from build123d import *

# Parameters (mm, degrees)
SKETCH010_R           = 35
PAD001_DEPTH          = 1
SKETCH011_R           = 4
PAD002_DEPTH          = 12
POLARPATTERN003_COUNT = 3
SKETCH012_R           = 1.88
POCKET004_DEPTH       = 212.690759
POLARPATTERN004_COUNT = 3
SKETCH013_R           = 5.15
POCKET005_DEPTH       = 1.001
BODY003_ROLL_ANGLE    = 180
BODY003_PITCH_ANGLE   = 60


with BuildPart() as part:
    # Sketch010 → Pad001 (new body)
    with BuildSketch(Plane.XZ):
        Circle(SKETCH010_R)
    extrude(amount=PAD001_DEPTH)

    # Sketch011 (on Face3 of Pad001) → Pad002 (join)
    with BuildSketch(Plane.XZ.offset(1)):
        with Locations((0, 30)):
            Circle(SKETCH011_R)
    pad002 = extrude(amount=PAD002_DEPTH)

    # PolarPattern003: Pad002 ×3 about axis
    polarpattern003_axis = Axis((0, -1, 0), (0, -1, 0))
    for i in range(1, POLARPATTERN003_COUNT):
        add(pad002.rotate(polarpattern003_axis, i * 360 / POLARPATTERN003_COUNT))

    # Sketch012 (on Face8 of PolarPattern003) → Pocket004 (cut, through all)
    with BuildSketch(Plane.XZ.offset(13)):
        with Locations((0, 30)):
            Circle(SKETCH012_R)
    pocket004 = extrude(amount=-POCKET004_DEPTH, mode=Mode.SUBTRACT)

    # PolarPattern004: Pocket004 ×3 about axis
    polarpattern004_axis = Axis((0, -13, 0), (0, -1, 0))
    for i in range(1, POLARPATTERN004_COUNT):
        add(pocket004.rotate(polarpattern004_axis, i * 360 / POLARPATTERN004_COUNT), mode=Mode.SUBTRACT)

    # Sketch013 (on Face3 of PolarPattern004) → Pocket005 (cut, through all)
    with BuildSketch(Plane.XZ.offset(1)):
        Circle(SKETCH013_R)
    extrude(amount=-POCKET005_DEPTH, mode=Mode.SUBTRACT)


with BuildPart() as part_1:
    # Body003 roll: moved
    add(part.part.rotate(Axis((0, 0, 0), (1, 0, 0)), BODY003_ROLL_ANGLE))


with BuildPart() as part_2:
    # Body003 pitch: moved
    add(part_1.part.rotate(Axis((0, 0, 0), (0, 1, 0)), BODY003_PITCH_ANGLE))


with BuildPart() as part_3:
    # Body003 placement: moved
    add(part_2.part.moved(Location((75.34421, -18, 43.5))))


solid = part_3.part
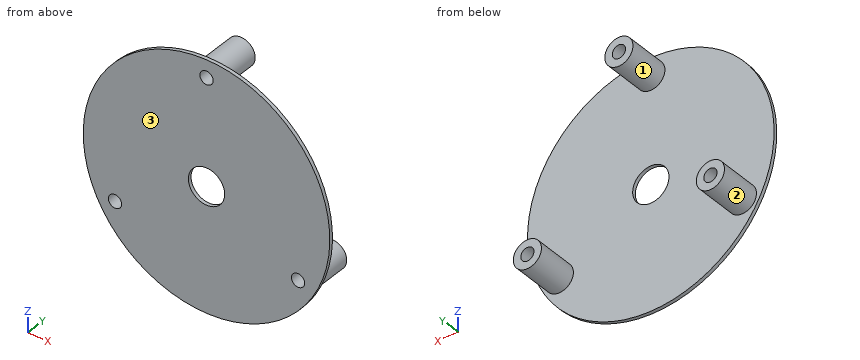
Design review of the part built by this model. Coordinates are the model's own, in mm. Face numbers are marked on the shaded views. Coordinates: 2 decimals unless noted, no trailing zeros. Loops run counter-clockwise (first coordinate to the right, second up) from the corner with the lowest first, then second, coordinate; pieces in that order, holes last. Notation, with made-up numbers: (-39.75, 44) - (-0.75, 44) arc R9 cw to (-0.75, 61) - close; hole circle Ø4 at (17.25, 60.25). An arc over 180 degrees is marked (long way). Use CSV: the item, a comma, the result in double quotes. Start each with the question number.
1. Add section D-D on z = 43.5. Give the boundary of the cut face in (x, y).
2. Add section A-A on z = 73.5. Give the boundary of the cut face in (x, y).
3. Clearance check with flat-ended pins moving along their axes: pin 1 (5 mm diameter, centred on x = 56.5, z = 47.5, fed in from +Y); pin 2 (3 mm diameter, centred on y = -13, z = 69.5, fed in from +X); pin 3 (3.5 mm diameter, centred on x = 49.36, z = 28.5, fed in from +Y); pin 4 (5 mm diameter, centred on x = 101.32, z = 28.5, fed in from -Y). State where each tip first meets the part, or that it passes through.
4. To check wall thickness, follow probe 1 along X at (y, z) = (-10.75, 30); probe 2 along Y at (x, z) = (82, 69); probe 3 along Z at (x, y) = (100.5, -8.5). State the ranges of each line that lie inside material, in increasing order.
5. Mouldability with a two-part tool opening along X and no side actions: class the marked faces 1, 2 and 3 as released by +X, released by -X, zero draft, split by the parting line, or undercut.
6. Add section C-C on y = -15. Give the boundary of the cut face in (x, z).
7. Add section B-B on z = 28.5. Give the boundary of the cut face in (x, y), plus the area to 3 significant figures.
Resolved:
1,outline,"(40.34, -18) - (70.19, -18) - (70.19, -17) - (40.34, -17) - close; (80.49, -18) - (110.34, -18) - (110.34, -17) - (80.49, -17) - close"
2,outline,"(57.32, -18) - (73.46, -18) - (73.46, -5) - (71.34, -5) - (71.34, -17) - (57.32, -17) - close; (77.22, -18) - (93.37, -18) - (93.37, -17) - (79.34, -17) - (79.34, -5) - (77.22, -5) - close"
3,pin 1,"y = -17"
3,pin 2,"x = 78.47"
3,pin 3,"through"
3,pin 4,"y = -18"
4,probe 1,"45.66 to 48.23, 50.5 to 53.07, 97.62 to 100.19, 102.46 to 105.03"
4,probe 2,"-18 to -17"
4,probe 3,"24.59 to 26.81, 30.19 to 32.41"
5,face 1,"split by the parting line"
5,face 2,"undercut"
5,face 3,"zero draft"
6,outline,"circle Ø8 at (49.36, 28.5); circle Ø8 at (75.34, 73.5); circle Ø8 at (101.32, 28.5); hole circle Ø3.76 at (49.36, 28.5); hole circle Ø3.76 at (75.34, 73.5); hole circle Ø3.76 at (101.32, 28.5)"
7,outline,"(43.72, -18) - (47.48, -18) - (47.48, -5) - (45.36, -5) - (45.36, -17) - (43.72, -17) - close; (51.24, -18) - (99.44, -18) - (99.44, -5) - (97.32, -5) - (97.32, -17) - (53.36, -17) - (53.36, -5) - (51.24, -5) - close; (103.2, -18) - (106.97, -18) - (106.97, -17) - (105.32, -17) - (105.32, -5) - (103.2, -5) - close"
7,area,"157 mm2"
